from build123d import *

# Parameters (mm, degrees)
CROQUIS1_W              = 1300
CROQUIS1_H              = 145
SALIENTE_EXTRUIR1_DEPTH = 35
CROQUIS2_W              = 35
CROQUIS2_H              = 145
CORTAR_EXTRUIR1_DEPTH   = 600
CROQUIS3_W              = 35
CROQUIS3_H              = 65
SALIENTE_EXTRUIR2_DEPTH = 50


with BuildPart() as part:
    # Croquis1 → Saliente-Extruir1 (new body)
    with BuildSketch(Plane.XY):
        Rectangle(CROQUIS1_W, CROQUIS1_H)
    extrude(amount=SALIENTE_EXTRUIR1_DEPTH)

    # Croquis2 → Cortar-Extruir1 (cut)
    with BuildSketch(Plane.ZY.offset(650)):
        with Locations((17.5, 0)):
            Rectangle(CROQUIS2_W, CROQUIS2_H)
    extrude(amount=-CORTAR_EXTRUIR1_DEPTH, mode=Mode.SUBTRACT)

    # Croquis3 → Saliente-Extruir2 (add)
    with BuildSketch(Plane.ZY.offset(50)):
        with Locations((17.5, 0)):
            Rectangle(CROQUIS3_W, CROQUIS3_H)
    extrude(amount=SALIENTE_EXTRUIR2_DEPTH)


solid = part.part
Geometry check sheet. Reference: the model listing, model coordinates, mm. A direction names the side the tool comes from. Round coordinates to 2 decimals unless told otherwise and drop trailing zeros. Loops run counter-clockwise (first coordinate to the right, second up) from the corner with the lowest first, then second, coordinate; pieces in that order, holes last. Notation, with made-up numbers: (-32.75, 46) - (-10.75, 46) arc R21 cw to (-10.75, 78) - close; hole circle Ø7 at (-8.5, 59). An arc over 180 degrees is marked (long way). One line per question, with ' | ' between items. Start each with the question number.
1. Depth check by flat-ended pin: pin 1 (10.5 mm diameter, centred on x = -66, z = 19.5, fed in from +Y); pin 2 (1.5 mm diameter, centred on x = 419.5, y = 47, fed in from -Z); pin 3 (1.5 mm diameter, centred on y = -50, z = 19.5, fed in from -X); pin 4 (17.5 mm diameter, centred on x = -79.5, z = 21.5, fed in from -Y). Enter the tip coordinate at first touch or a pass-through.
2. Cross-section at A-A on z = 16. Record the cut outline in (x, y), then the cut area to 3 significant figures.
3. Draft check along Y on faces 4 (the face through (270, 1, 0)), 5 (the face through (-75, 32.5, 17)), 6 (the face through (-75, -32.5, 17)). Enter one of: released by +Y, released by -Y, zero draft, split by the parting line, or undercut.
4. Tool access check on faces 1 (the face through (-50, -52, 17)), 2 (the face through (650, -1, 17)), 3 (the face through (-50, 53, 17)). Record the directions out of +Z, -Z, +X, -X, +Y, -Y that give a thin tool (end or side, any length) a straight path to the whole face; none if there is none.
5. Scan line: line 1 (X direction, y = 42, z = 20.5). Record every from-to range of solid material in increasing order. Write a range as [from, to].
6. Cross-section at B-B on y = -43. Record the cut outline in (x, z).
Taken from the geometry:
1) pin 1: y = 32.5 | pin 2: z = 0 | pin 3: x = -50 | pin 4: y = -32.5
2) outline: (-100, -32.5) - (-50, -32.5) - (-50, -72.5) - (650, -72.5) - (650, 72.5) - (-50, 72.5) - (-50, 32.5) - (-100, 32.5) - close | area: 105,000 mm²
3) face 4: zero draft | face 5: released by +Y | face 6: released by -Y
4) face 1: +Z, -Z, -X, -Y | face 2: +Z, -Z, +X, +Y, -Y | face 3: +Z, -Z, -X, +Y
5) line 1: [-50, 650]
6) outline: (-50, 0) - (650, 0) - (650, 35) - (-50, 35) - close
